from build123d import *

# Parameters (mm, degrees)
CROQUIS1_W              = 3
CROQUIS1_H              = 3
SALIENTE_EXTRUIR1_DEPTH = 3


with BuildPart() as part:
    # Croquis1 → Saliente-Extruir1 (new body)
    with BuildSketch(Plane.XY):
        with BuildLine():
            Line((-30, -11.425), (-30, -8.425))
            Line((-30, -8.425), (-1.5, -8.425))
            Line((-1.5, -8.425), (-1.5, 30))
            Line((-1.5, 30), (-1.5, 33))
            Line((-1.5, 33), (-13, 33))
            ThreePointArc((-13, 33), (-27.142135624, 27.142135624), (-33, 13))
            Line((-33, 13), (-33, -13))
            ThreePointArc((-33, -13), (-27.142135624, -27.142135624), (-13, -33))
            Line((-13, -33), (13, -33))
            ThreePointArc((13, -33), (27.142135624, -27.142135624), (33, -13))
            Line((33, -13), (33, 13))
            ThreePointArc((33, 13), (27.142135624, 27.142135624), (13, 33))
            Line((13, 33), (1.5, 33))
            Line((1.5, 33), (1.5, 30))
            Line((1.5, 30), (1.5, -8.425))
            Line((1.5, -8.425), (30, -8.425))
            Line((30, -8.425), (30, -11.425))
            Line((30, -11.425), (1.5, -11.425))
            Line((1.5, -11.425), (1.5, -30))
            Line((1.5, -30), (-1.5, -30))
            Line((-1.5, -30), (-1.5, -11.425))
            Line((-1.5, -11.425), (-30, -11.425))
        make_face()
        with Locations((-23.5, -16.2)):
            Rectangle(CROQUIS1_W, CROQUIS1_H, mode=Mode.SUBTRACT)
        with Locations((-12.5, -16.2)):
            Rectangle(CROQUIS1_W, CROQUIS1_H, mode=Mode.SUBTRACT)
        with Locations((12.5, -16.2)):
            Rectangle(CROQUIS1_W, CROQUIS1_H, mode=Mode.SUBTRACT)
        with Locations((23.5, -16.2)):
            Rectangle(CROQUIS1_W, CROQUIS1_H, mode=Mode.SUBTRACT)
        with Locations((-5.5, 16.4)):
            Rectangle(CROQUIS1_W, CROQUIS1_H, mode=Mode.SUBTRACT)
        with Locations((5.5, 16.4)):
            Rectangle(CROQUIS1_W, CROQUIS1_H, mode=Mode.SUBTRACT)
    extrude(amount=SALIENTE_EXTRUIR1_DEPTH)


solid = part.part
The listing builds one solid part. Answer for the finished solid, in the listing's coordinates (mm). A direction names the side the tool comes from. Coordinates: 2 decimals unless noted, no trailing zeros. Loops run counter-clockwise (first coordinate to the right, second up) from the corner with the lowest first, then second, coordinate; pieces in that order, holes last.
1) Find the intervals of material crossed by L1, parallel to Y at x = -5, z = 1.6 (3 decimals); L2, parallel to Y at x = 2.5, z = 1 (3 decimals); L3, parallel to Y at x = 11.5, z = 1.2 (3 decimals), in increasing order.
2) Find section C-C on x = -28.5. Write down the section's boundary in (y, z) (3 decimals), then the cut area to 3 significant figures.
3) Find section B-B on x = -5. Write down the section's boundary in (y, z) (3 decimals), then the cut area to 3 significant figures.
4) Find section A-A on y = -7. Write down the section's boundary in (x, z).
5) A tool of negligible diameter and unlimited length cuts with its end or side. For faces 1 (the face through (-1.5, 12, 1)), 2 (the face through (12, -17.7, 1)), 3 (the face through (-8, 0, 3)), from which of +Z, -Z, +X, -X, +Y, -Y can it reach the whole face along a straight path? Write none if from no direction.
6) Flat-ended cylindrical pins translate along their axes: pin 1 Ø0.9 at (y, z) = (-16, 1.5) entering from -X; pin 2 Ø0.9 at (x, z) = (-23, 1.5) entering from +Y. Find the tip coordinate at first contact, or state that the pin passes through.
7) Find section D-D on z = 2.5. Give the number of separate pieces and of enclosed holes in the cut face, then the cut area to 3 significant figures.
Values:
1. L1: y = -33 to -11.425, -8.425 to 14.9, 17.9 to 33
1. L2: y = -33 to -11.425, -8.425 to 33
1. L3: y = -33 to -17.7, -14.7 to -11.425, -8.425 to 33
2. outline: (-25.639, 0) - (-11.425, 0) - (-11.425, 3) - (-25.639, 3) - close; (-8.425, 0) - (25.639, 0) - (25.639, 3) - (-8.425, 3) - close
2. area: 145 mm2
3. outline: (-33, 0) - (-11.425, 0) - (-11.425, 3) - (-33, 3) - close; (-8.425, 0) - (14.9, 0) - (14.9, 3) - (-8.425, 3) - close; (17.9, 0) - (33, 0) - (33, 3) - (17.9, 3) - close
3. area: 180 mm2
4. outline: (-33, 0) - (-1.5, 0) - (-1.5, 3) - (-33, 3) - close; (1.5, 0) - (33, 0) - (33, 3) - (1.5, 3) - close
5. face 1: +Z, -Z, +Y
5. face 2: +Z, -Z
5. face 3: +Z, +X, -X, +Y, -Y
6. pin 1: stops at x = -32.84
6. pin 2: stops at y = 30.57
7. separate pieces: 1
7. enclosed holes: 6
7. area: 3,600 mm2
